Could you check a few things on this model? Use its own coordinates, in mm. A direction names the side the tool comes from. Round coordinates to 2 decimals unless told otherwise and drop trailing zeros. Write each loop counter-clockwise with the first axis right and the second up, starting at its lowest first coordinate (ties: lowest second). Pieces come first, ordered by that corner, then holes. Notation, with made-up numbers: M -12.75,85.5 L 29.25,85.5 A5 ccw 29.25,90.5 Z; hole C 69.5,65.25 d6. An arc over 180 degrees is marked long. One line per question, with ' | ' between items. Start each with the question number.
```python
from build123d import *

# Parameters (mm, degrees)
SKETCH_1_R             = 1.6
SM_BASE_FLANGE_1_DEPTH = 0.3
OTHER_START            = -4
OTHER_1_OUTLINE_W      = 3
OTHER_1_OUTLINE_H      = 0.3
OTHER_1_DEPTH          = 8.959734012
OTHER_START_2          = 4.659734012
OTHER_1_2_OUTLINE_R    = 1.6
OTHER_1_2_DEPTH        = 1.0366
OTHER_1_3_DEPTH        = 8


with BuildPart() as part:
    # 基体-法兰1: sheet metal written as solids
    # Sketch 1 → 基体-法兰1 (new body)
    with BuildSketch(Plane(origin=(0, 0, 0), x_dir=(1, 0, 0), z_dir=(0, 1, 0))):
        with BuildLine():
            Line((-1.5, -8), (-1.5, -2.598076211))
            ThreePointArc((-1.5, -2.598076211), (0, 3), (1.5, -2.598076211))
            Line((1.5, -2.598076211), (1.5, -8))
            ThreePointArc((1.5, -8), (0, -9.5), (-1.5, -8))
        make_face()
        with Locations(Location((0, 0, 0), (0, 0, 270))):
            Circle(SKETCH_1_R, mode=Mode.SUBTRACT)
        with BuildLine():
            Line((0.6, -6.7), (0.6, -8))
            ThreePointArc((0.6, -8), (0, -8.6), (-0.6, -8))
            Line((-0.6, -8), (-0.6, -6.7))
            ThreePointArc((-0.6, -6.7), (0, -6.1), (0.6, -6.7))
        make_face(mode=Mode.SUBTRACT)
    extrude(amount=-SM_BASE_FLANGE_1_DEPTH)

    # Other 1: read off the stored shape, not the designer's step
    # Other 1 outline → Other 1 (cut)
    with BuildSketch(Plane.XY.offset(OTHER_START)):
        with Locations((0, -0.15)):
            Rectangle(OTHER_1_OUTLINE_W, OTHER_1_OUTLINE_H)
    extrude(amount=OTHER_1_DEPTH, mode=Mode.SUBTRACT)

    # Other 1 2 outline → Other 1 2 (add)
    with BuildSketch(Plane.XY.offset(OTHER_START_2)):
        with BuildLine():
            ThreePointArc((1.5, 2.442189777), (0, 8.040265988), (-1.5, 2.442189777))
            Line((-1.5, 2.442189777), (-1.5, 0))
            Line((-1.5, 0), (1.5, 0))
            Line((1.5, 0), (1.5, 2.442189777))
        make_face()
        with Locations((0, 5.040265988)):
            Circle(OTHER_1_2_OUTLINE_R, mode=Mode.SUBTRACT)
    extrude(amount=OTHER_1_2_DEPTH)

    # Other 1 3 outline → Other 1 3 (cut)
    with BuildSketch(Plane.YZ.offset(OTHER_START)):
        with BuildLine():
            Line((0.7366, 4.959734012), (10, 4.959734012))
            Line((10, 4.959734012), (10, 5.696334012))
            Line((10, 5.696334012), (0, 5.696334012))
            ThreePointArc((0, 5.696334012), (0.215745145, 5.175479157), (0.7366, 4.959734012))
        make_face()
        with BuildLine():
            Line((10, -4), (10, 4.659734016))
            Line((10, 4.659734016), (0.7366, 4.659734012))
            ThreePointArc((0.7366, 4.659734012), (0.00361311, 4.963347123), (-0.3, 5.696334012))
            Line((-0.3, 5.696334012), (-0.3, 7))
            Line((-0.3, 7), (-2, 7))
            Line((-2, 7), (-2, -4))
            Line((-2, -4), (10, -4))
        make_face()
    extrude(amount=OTHER_1_3_DEPTH, mode=Mode.SUBTRACT)


solid = part.part
```
1. Suppose I cut it at D-D (y = 4.5). Write out the boundary of the cut face in (x, z).
2. Suppose I cut it at B-B (y = 6.5). Write out the boundary of the cut face in (x, z).
3. Suppose I cut it at C-C (x = -1). Write out the boundary of the cut face in (y, z).
4. Which directions (+Z, -Z, +X, -X, +Y, -Y) give clear straight access to the entire face, cutting with the end or side of a thin tool? Please do faces 1 (the face through (-1.4, 3.5, 4.96)), 2 (the face through (-1, -0.3, 8)).
5. I'm going to push flat-ended pins straight in: P1, Ø1.8, axis at x = 0, y = 4.5, coming from the +Z side; P2, Ø1.5, axis at x = 0.5, z = 7.5, coming from the +Y side; P3, Ø3, axis at x = 1, y = 5.5, coming from the +Z side. Where does each tip first touch, or does it pass through?
6. Suppose I cut it at A-A (x = 0). Write out the boundary of the cut face in (y, z), and give its area (3 significant figures).
7. I need wall thicknesses on line 1 along Y through (x, z) = (1.2, 7.9); line 2 along Z through (x, y) = (1.2, 3); line 3 along Y through (x, z) = (0, 4.8). Which ranges of each line are inside material? Lowest first, please. Write a range as from..to.
Computed:
1) outline: M -2.95,4.66 L -1.51,4.66 L -1.51,4.96 L -2.95,4.96 Z; M 1.51,4.66 L 2.95,4.66 L 2.95,4.96 L 1.51,4.96 Z
2) outline: M -2.62,4.66 L -0.66,4.66 L -0.66,4.96 L -2.62,4.96 Z; M 0.66,4.66 L 2.62,4.66 L 2.62,4.96 L 0.66,4.96 Z
3) outline: M -0.3,5.7 A1.04 ccw 0.74,4.66 L 3.79,4.66 L 3.79,4.96 L 0.74,4.96 A0.74 cw 0,5.7 L 0,9.12 L -0.3,9.12 Z; M 6.29,4.66 L 7.87,4.66 L 7.87,4.96 L 6.29,4.96 Z
4) face 1: +Z, +X, -X, +Y | face 2: +Z, -Z, +X, -X, -Y
5) P1: passes through | P2: stops at y = 0 | P3: stops at z = 4.96
6) outline: M -0.3,5.7 A1.04 ccw 0.74,4.66 L 3.44,4.66 L 3.44,4.96 L 0.74,4.96 A0.74 cw 0,5.7 L 0,6.1 L -0.3,6.1 Z; M -0.3,8.6 L 0,8.6 L 0,9.5 L -0.3,9.5 Z; M 6.64,4.66 L 8.04,4.66 L 8.04,4.96 L 6.64,4.96 Z | area: 2.04 mm²
7) line 1: y = -0.3..0 | line 2: z = 4.66..4.96 | line 3: y = 0.22..3.44, 6.64..8.04
